from build123d import *

# Parameters (mm, degrees)
F1_DEPTH = 5
F3_DEPTH = 15
F4_DEPTH = 50


with BuildPart() as f1:
    # F0 (on Front) → F1 (new body)
    with BuildSketch(Plane.XZ):
        with BuildLine():
            Line((0, -41.3114728638), (0, 38.6885271362))
            Line((0, 38.6885271362), (-53, 38.6885271362))
            ThreePointArc((-53, 38.6885271362), (-51.2309986969, -4.1091349892), (-30, -41.3114728638))
            Line((-30, -41.3114728638), (0, -41.3114728638))
        make_face()
    extrude(amount=F1_DEPTH)

    # F2 (on face) → F3 (join)
    with BuildSketch(Plane.XY.offset(38.6885271362)):
        with BuildLine():
            Line((-6.3985955209, 0), (-1.165957073, 0))
            ThreePointArc((-1.165957073, 0), (-3.782276297, 1.118718873), (-6.3985955209, 0))
        make_face()
        with BuildLine():
            ThreePointArc((-6.3985955209, -5), (-3.782276297, -6.118718873), (-1.165957073, -5))
            Line((-1.165957073, -5), (-6.3985955209, -5))
        make_face()
    extrude(amount=-F3_DEPTH)

    # F2 (on face) → F4 (join)
    with BuildSketch(Plane.XY.offset(38.6885271362)):
        with BuildLine():
            ThreePointArc((-1.165957073, -5), (-0.4234930325, -3.8467372662), (-0.163557424, -2.5))
            ThreePointArc((-0.163557424, -2.5), (-0.4234930325, -1.1532627338), (-1.165957073, 0))
            Line((-1.165957073, 0), (-6.3985955209, 0))
            ThreePointArc((-6.3985955209, 0), (-7.40099517, -2.5), (-6.3985955209, -5))
            Line((-6.3985955209, -5), (-1.165957073, -5))
        make_face()
        with BuildLine():
            Line((-6.3985955209, 0), (-1.165957073, 0))
            ThreePointArc((-1.165957073, 0), (-3.782276297, 1.118718873), (-6.3985955209, 0))
        make_face()
        with BuildLine():
            ThreePointArc((-6.3985955209, -5), (-3.782276297, -6.118718873), (-1.165957073, -5))
            Line((-1.165957073, -5), (-6.3985955209, -5))
        make_face()
    extrude(amount=F4_DEPTH)


solid = f1.part
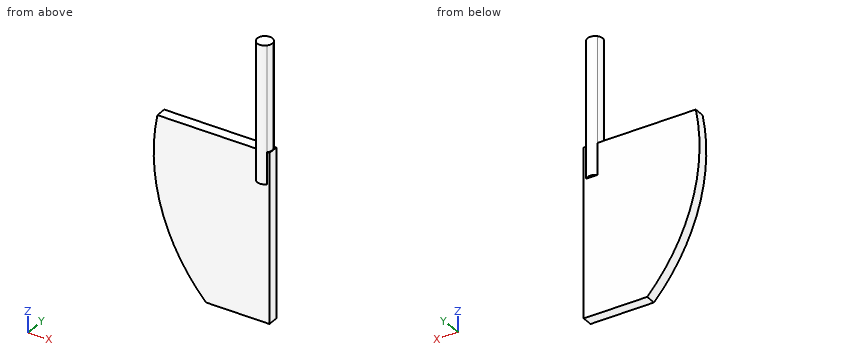
Geometry check sheet. Reference: the model listing, model coordinates, mm. Give positions to 0.01 mm unless a question says otherwise; leave off trailing zeros. Write each loop counter-clockwise with the first axis right and the second up, starting at its lowest first coordinate (ties: lowest second). Pieces come first, ordered by that corner, then holes. Notation, with made-up numbers: (53.25, 51.25) - (110.25, 51.25) arc R29 cw to (110.25, 84.25) - close; hole circle Ø4 at (9.5, -36.75). An arc over 180 degrees is marked (long way). Put each result on its own line as item: value.
1. Sectioned sample at A-A, the plane z = 74.5. Enter the section's corners in (x, y).
Ans:
outline: circle Ø7.24 at (-3.78, -2.5)
2. Sectioned sample at D-D, the plane x = -32. Enter the section's corners in (y, z).
Ans:
outline: (-5, -39.12) - (0, -39.12) - (0, 38.69) - (-5, 38.69) - close
3. Sectioned sample at B-B, the plane x = -9. Enter the section's corners in (y, z), plus the area to 3 significant figures.
Ans:
outline: (-5, -41.31) - (0, -41.31) - (0, 38.69) - (-5, 38.69) - close
area: 400 mm²
4. Go/stop test with flat-tipped pins: pin 1 (0.6 mm diameter, centred on x = -3, y = 0.5, fed in from -Z); pin 2 (3 mm diameter, centred on y = -4, z = 28.5, fed in from +X); pin 3 (2 mm diameter, centred on x = -21, y = -4.5, fed in from +Z); pin 4 (16.5 mm diameter, centred on x = -38, z = -6.5, fed in from -Y). Record where each tip stops, or that it passes through.
Ans:
pin 1: stops at z = 23.69
pin 2: stops at x = 0
pin 3: stops at z = 38.69
pin 4: stops at y = -5
5. Thickness scan on line 1 (Y direction, x = -33, z = -18.5); line 2 (X direction, y = -2.75, z = 74); line 3 (Z direction, x = -24, y = -1.5). Record the ranges inside material, lowest first.
Ans:
line 1: y = -5 to 0
line 2: x = -7.39 to -0.17
line 3: z = -41.31 to 38.69
6. Sectioned sample at C-C, the plane z = 26. Enter the section's corners in (x, y).
Ans:
outline: (-54.62, -5) - (-6.4, -5) arc R3.62 ccw to (-1.17, -5) - (0, -5) - (0, 0) - (-1.17, 0) arc R3.62 ccw to (-6.4, 0) - (-54.62, 0) - close
